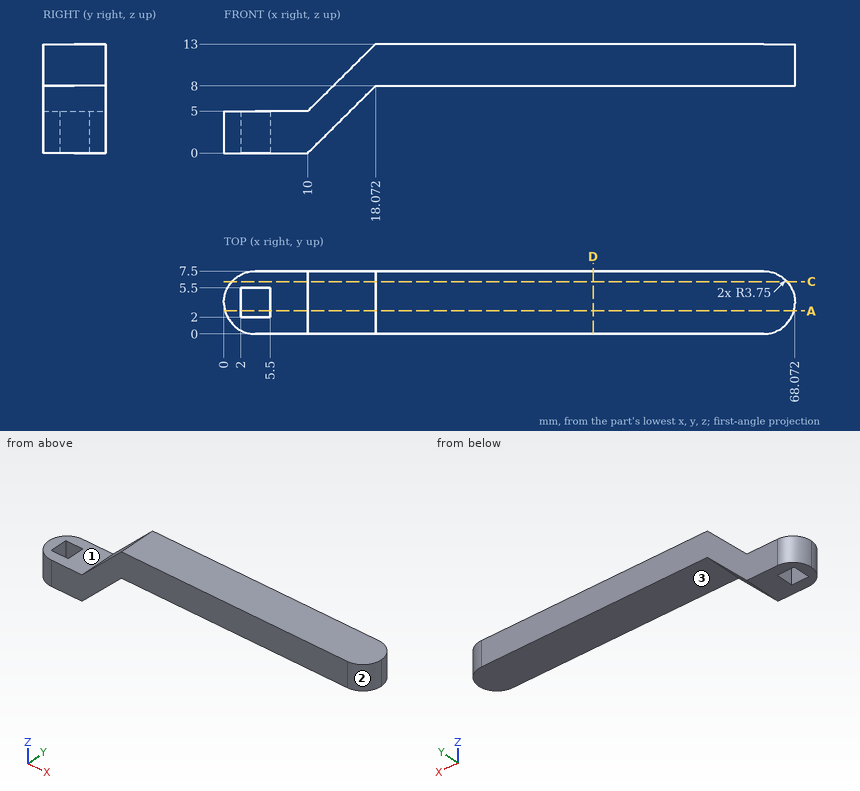
Could you check a few things on this drawing? It's one solid part, dimensions in mm from its lowest x, y, z. A direction names the side the tool comes from. Give positions to 0.01 mm unless a question says otherwise; leave off trailing zeros. Write each loop counter-clockwise with the first axis right and the second up, starting at its lowest first coordinate (ties: lowest second). Pieces come first, ordered by that corner, then holes. Notation, with made-up numbers: (-2, -31) -> (8, -31) arc R14 ccw to (8, -8) -> close; hole circle Ø1 at (70.25, 8). An arc over 180 degrees is marked (long way). Answer as a JSON object with one key per item and string values.
Q1. Suppose I cut it at C-C on y = 6.25. Write out the boundary of the cut face in (x, z) (1 decimal), then the cut area to 3 significant figures.
Taken from the geometry:
{"outline": "(1, 0) -> (10, 0) -> (18.1, 8) -> (67.1, 8) -> (67.1, 13) -> (18.1, 13) -> (10, 5) -> (1, 5) -> close", "area": "331 mm²"}
Q2. Suppose I cut it at A-A on y = 2.75. Write out the boundary of the cut face in (x, z).
Taken from the geometry:
{"outline": "(0.14, 0) -> (2, 0) -> (2, 5) -> (0.14, 5) -> close; (5.5, 0) -> (10, 0) -> (18.07, 8) -> (67.94, 8) -> (67.94, 13) -> (18.07, 13) -> (10, 5) -> (5.5, 5) -> close"}
Q3. Suppose I cut it at D-D on x = 44. Write out the boundary of the cut face in (y, z), then the cut area to 3 significant figures.
Taken from the geometry:
{"outline": "(0, 8) -> (7.5, 8) -> (7.5, 13) -> (0, 13) -> close", "area": "37.5 mm²"}
Q4. Will these pins go through, and if not, where does the flat tip stop? pin 1 Ø1 at (y, z) = (3, 9.5) entering from -X (1 decimal); pin 2 Ø4 at (x, y) = (40.5, 3) entering from -Z; pin 3 Ø3 at (y, z) = (3.5, 3) entering from +X.
Taken from the geometry:
{"pin 1": "stops at x = 14", "pin 2": "stops at z = 8", "pin 3": "stops at x = 14.54"}
Q5. Which directions (+Z, -Z, +X, -X, +Y, -Y) give clear straight access to the entire face, cutting with the end or side of a thin tool? Please do the marked faces 1, 2 and 3.
Taken from the geometry:
{"face 1": "+Z, -X, +Y, -Y", "face 2": "+Z, -Z, +X, -Y", "face 3": "-Z, +X, +Y, -Y"}
Q6. Please list where these lines run through material, in increasing order: L1, parallel to Z at x = 55.5, y = 3.5; L2, parallel to X at y = 3.5, z = 3.5; L3, parallel to X at y = 4, z = 4 (1 decimal).
Taken from the geometry:
{"L1": "z = 8 to 13", "L2": "x = 0.01 to 2, 5.5 to 13.53", "L3": "x = 0 to 2, 5.5 to 14"}
